from build123d import *

# Parameters (mm, degrees)
SKETCH1_R           = 41.1
BOSS_EXTRUDE1_DEPTH = 4.5
SKETCH5_R           = 38.4
BOSS_EXTRUDE3_DEPTH = 0.5
SKETCH2_R           = 11
SKETCH2_R_2         = 4.5
CUT_EXTRUDE1_DEPTH  = 4
SKETCH3_R           = 7.5
CUT_EXTRUDE2_DEPTH  = 59.261651195
FILLET1_R           = 4


with BuildPart() as part:
    # Sketch1 → Boss-Extrude1 (new body)
    with BuildSketch(Plane(origin=(0, 0, 0), x_dir=(1, 0, 0), z_dir=(0, 1, 0))):
        with Locations(Location((0, 0, 0), (0, 0, 270))):
            Circle(SKETCH1_R)
    extrude(amount=BOSS_EXTRUDE1_DEPTH)

    # Sketch5 → Boss-Extrude3 (add)
    with BuildSketch(Plane.XZ):
        with Locations(Location((0, 0, 0), (0, 0, 270))):
            Circle(SKETCH5_R)
    extrude(amount=BOSS_EXTRUDE3_DEPTH)

    # Sketch2 → Cut-Extrude1 (cut)
    # profile 1 of 2: a face of its own
    with BuildSketch(Plane(origin=(0, 4.5, 0), x_dir=(1, 0, 0), z_dir=(0, 1, 0))):
        with Locations(Location((0, 0, 0), (0, 0, 270))):
            Circle(SKETCH2_R)
        Circle(SKETCH2_R_2, mode=Mode.SUBTRACT)
    # profile 2 of 2: a face of its own
    with BuildSketch(Plane(origin=(0, 4.5, 0), x_dir=(1, 0, 0), z_dir=(0, 1, 0))):
        Circle(SKETCH2_R_2)
    extrude(amount=-CUT_EXTRUDE1_DEPTH, mode=Mode.SUBTRACT)

    # Sketch3 → Cut-Extrude2 (cut, through all)
    with BuildSketch(Plane(origin=(0, 0.5, 0), x_dir=(1, 0, 0), z_dir=(0, 1, 0))):
        with Locations(Location((0, 0, 0), (0, 0, 270))):
            Circle(SKETCH3_R)
    extrude(amount=-CUT_EXTRUDE2_DEPTH, mode=Mode.SUBTRACT)

    # Fillet1
    fillet1_edges = [part.edges().sort_by_distance(p)[0] for p in [
        (0, 4.5, -41.1),
    ]]
    fillet(fillet1_edges, radius=FILLET1_R)


solid = part.part
Read the model definition and answer for the solid it produces. Units are mm, in the model's axes. A direction names the side the tool comes from. Give positions to 0.01 mm unless a question says otherwise; leave off trailing zeros. Write each loop counter-clockwise with the first axis right and the second up, starting at its lowest first coordinate (ties: lowest second). Pieces come first, ordered by that corner, then holes. Notation, with made-up numbers: (58.5, 75) - (74.5, 75) arc R33 cw to (74.5, 111) - close; hole circle Ø9 at (-37.5, 37.5). An arc over 180 degrees is marked (long way). Answer in a Markdown table with one row per item. Add a question column.
Item 1: Flat-ended cylindrical pins translate along their axes: P1, Ø17.5, axis at x = 0, z = 0, coming from the +Y side; P2, Ø3, axis at y = 0, z = 30, coming from the +X side; P3, Ø1.5, axis at y = 2.5, z = 20, coming from the -X side; P4, Ø12, axis at x = 0, z = 0, coming from the +Y side. Find the tip coordinate at first contact, or state that the pin passes through.
Item 2: Section A-A, the plane z = 0 is taken. Write down the section's boundary in (x, y), and give its area (3 significant figures).
Item 3: Section C-C, the plane y = 2.95 is taken. Write down the section's boundary in (x, z).
Item 4: A tool of negligible diameter and unlimited length cuts with its end or side. For faces 1 (the face through (9, 4.5, 8)), 2 (the face through (2.6, 0.5, 7.2)), from which of +Z, -Z, +X, -X, +Y, -Y can it reach the whole face along a straight path? Write none if from no direction.
Item 5: Section B-B, the plane x = 0 is taken. Write down the section's boundary in (y, z), and give its area (3 significant figures).
Item 6: Find the intervals of material crossed by L1, parallel to X at y = -0.15, z = 0; L2, parallel to Z at x = -6, y = 2.6; L3, parallel to Y at x = -28, z = -24.5, in increasing order.
Item 7: Determine the mould class of faces 3 (the face through (32.38, -0.25, -20.64)), 4 (the face through (0.33, 0.007, -7.493)), 5 (the face through (37, 0, -12)) for opening direction Z: pulls with the +Z half, pulls with the -Z half, needs draft (parallel to the pull), parting line crosses it, or undercut.
Recorded:
| question | item | result |
|---|---|---|
| 1 | P1 | stops at y = 0.5 |
| 1 | P2 | stops at x = 29.61 |
| 1 | P3 | stops at x = -35.88 |
| 1 | P4 | passes through |
| 2 | outline | (-41.1, 0) - (-38.4, 0) - (-38.4, -0.5) - (-7.5, -0.5) - (-7.5, 0.5) - (-11, 0.5) - (-11, 4.5) - (-37.1, 4.5) arc R4 ccw to (-41.1, 0.5) - close; (7.5, -0.5) - (38.4, -0.5) - (38.4, 0) - (41.1, 0) - (41.1, 0.5) arc R4 ccw to (37.1, 4.5) - (11, 4.5) - (11, 0.5) - (7.5, 0.5) - close |
| 2 | area | 298 mm2 |
| 3 | outline | circle Ø80.52 at (0, 0); hole circle Ø22 at (0, 0) |
| 4 | face 1 | +Z, -Z, +X, -X, +Y |
| 4 | face 2 | +Y |
| 5 | outline | (-0.5, -38.4) - (0, -38.4) - (0, -41.1) - (0.5, -41.1) arc R4 ccw to (4.5, -37.1) - (4.5, -11) - (0.5, -11) - (0.5, -7.5) - (-0.5, -7.5) - close; (-0.5, 7.5) - (0.5, 7.5) - (0.5, 11) - (4.5, 11) - (4.5, 37.1) arc R4 ccw to (0.5, 41.1) - (0, 41.1) - (0, 38.4) - (-0.5, 38.4) - close |
| 5 | area | 298 mm2 |
| 6 | L1 | x = -38.4 to -7.5, 7.5 to 38.4 |
| 6 | L2 | z = -40.06 to -9.22, 9.22 to 40.06 |
| 6 | L3 | y = -0.5 to 4.5 |
| 7 | face 3 | parting line crosses it |
| 7 | face 4 | undercut |
| 7 | face 5 | needs draft |
